```python
from build123d import *

# Parameters (mm, degrees)
SKETCH1_W             = 27
SKETCH1_H             = 27
SKETCH1_W_2           = 21
SKETCH1_H_2           = 21
BOSS_EXTRUDE1_DEPTH   = 70
BOSS_EXTRUDE1_2_DEPTH = 70
SKETCH2_W             = 120
SKETCH2_H             = 25
BOSS_EXTRUDE2_DEPTH   = 10
SKETCH3_W             = 3
SKETCH3_H             = 25
BOSS_EXTRUDE3_DEPTH   = 27
SKETCH4_R             = 2.15
CUT_EXTRUDE1_DEPTH    = 38


with BuildPart() as part:
    # Sketch1 → Boss-Extrude1 (new body)
    with BuildSketch(Plane(origin=(0, 0, 0), x_dir=(1, 0, 0), z_dir=(0, 1, 0))):
        with Locations((13.5, 13.5)):
            Rectangle(SKETCH1_W, SKETCH1_H)
        with Locations((13.5, 13.5)):
            Rectangle(SKETCH1_W_2, SKETCH1_H_2, mode=Mode.SUBTRACT)
    extrude(amount=BOSS_EXTRUDE1_DEPTH)



with BuildPart() as body_2:
    # Sketch1 → Boss-Extrude1 2 (new body)
    with BuildSketch(Plane(origin=(0, 0, 0), x_dir=(1, 0, 0), z_dir=(0, 1, 0))):
        with Locations((-16.5, 13.5)):
            Rectangle(SKETCH1_W, SKETCH1_H)
        with Locations((-16.5, 13.5)):
            Rectangle(SKETCH1_W_2, SKETCH1_H_2, mode=Mode.SUBTRACT)
    extrude(amount=BOSS_EXTRUDE1_2_DEPTH)


with BuildPart() as part_1:
    add(part.part)

    add(body_2.part)  # Boss-Extrude2 merges body 2
    # Sketch2 → Boss-Extrude2 (add)
    with BuildSketch(Plane.XY):
        with Locations((-2, 35)):
            Rectangle(SKETCH2_W, SKETCH2_H)
    extrude(amount=BOSS_EXTRUDE2_DEPTH)

    # Sketch3 → Boss-Extrude3 (add)
    with BuildSketch(Plane(origin=(0, 0, -27), x_dir=(-1, 0, 0), z_dir=(0, 0, -1))):
        with Locations((1.5, 35)):
            Rectangle(SKETCH3_W, SKETCH3_H)
    extrude(amount=-BOSS_EXTRUDE3_DEPTH)

    # Sketch4 → Cut-Extrude1 (cut, through all)
    with BuildSketch(Plane(origin=(0, 0, -27), x_dir=(-1, 0, 0), z_dir=(0, 0, -1))):
        with Locations((-13.5, 60)):
            Circle(SKETCH4_R)
        with Locations((16.5, 60)):
            Circle(SKETCH4_R)
        with Locations((-13.5, 10)):
            Circle(SKETCH4_R)
        with Locations((16.5, 10)):
            Circle(SKETCH4_R)
    extrude(amount=-CUT_EXTRUDE1_DEPTH, mode=Mode.SUBTRACT)


solid = part_1.part
```
Model file for the job. Use its own axes, mm. A direction names the side the tool comes from. Coordinates: 2 decimals unless noted, no trailing zeros. Loops run counter-clockwise (first coordinate to the right, second up) from the corner with the lowest first, then second, coordinate; pieces in that order, holes last. Notation, with made-up numbers: (51, 79.25) -> (77, 79.25) arc R23 cw to (77, 107.25) -> close; hole circle Ø5 at (-31, 65). An arc over 180 degrees is marked (long way). Answer as a JSON object with one key per item and string values.
Q1. 3-axis set-ups, long thin cutter, end or side, ignore diameter. For faces 1 (the flat face through (-17, 35, -24)), 2 (the flat face through (0, 11, -13)), 3 (the flat face through (0, 59, -13)): which of +Z, -Z, +X, -X, +Y, -Y reach the whole face in a straight line?
Report:
{"face 1": "+Y, -Y", "face 2": "+Z, -Z, -Y", "face 3": "+Z, -Z, +Y"}
Q2. Flat gauge pins, fed straight in: P1, Ø10.5, axis at y = 35, z = -10.5, coming from the -X side; P2, Ø7, axis at y = 55, z = -10.5, coming from the +X side; P3, Ø3.5, axis at x = -16.5, y = 10, coming from the +Z side; P4, Ø11, axis at x = 16.5, y = 53.5, coming from the +Z side. Where does each tip first touch, or does it go through?
Report:
{"P1": "stops at x = -30", "P2": "stops at x = 27", "P3": "passes through", "P4": "stops at z = 0"}
Q3. Pull direction Z, two halves, no side cores. Call faces 4 (the flat face through (13, 35, -3)), 5 (the flat face through (-2, 47.5, 4)), 6 (the flat face through (-27, 35, -13)): released by +Z, released by -Z, zero draft, split by the parting line, or undercut.
Report:
{"face 4": "undercut", "face 5": "zero draft", "face 6": "undercut"}
Q4. Cut at C-C (y = 17). List the corners of the cut face in (x, z).
Report:
{"outline": "(-30, -27) -> (-3, -27) -> (-3, 0) -> (-30, 0) -> close; (0, -27) -> (27, -27) -> (27, 0) -> (0, 0) -> close; hole (-27, -24) -> (-6, -24) -> (-6, -3) -> (-27, -3) -> close; hole (3, -24) -> (24, -24) -> (24, -3) -> (3, -3) -> close"}
Q5. Cut at D-D (z = -19). List the corners of the cut face in (x, y), and give its area (3 significant figures).
Report:
{"outline": "(-30, 0) -> (-27, 0) -> (-27, 70) -> (-30, 70) -> close; (-6, 0) -> (-3, 0) -> (-3, 22.5) -> (0, 22.5) -> (0, 0) -> (3, 0) -> (3, 70) -> (0, 70) -> (0, 47.5) -> (-3, 47.5) -> (-3, 70) -> (-6, 70) -> close; (24, 0) -> (27, 0) -> (27, 70) -> (24, 70) -> close", "area": "915 mm2"}
Q6. Cut at A-A (x = 13.5). List the corners of the cut face in (y, z).
Report:
{"outline": "(0, -27) -> (7.85, -27) -> (7.85, -24) -> (0, -24) -> close; (0, -3) -> (7.85, -3) -> (7.85, 0) -> (0, 0) -> close; (12.15, -27) -> (57.85, -27) -> (57.85, -24) -> (12.15, -24) -> close; (12.15, -3) -> (57.85, -3) -> (57.85, 0) -> (47.5, 0) -> (47.5, 10) -> (22.5, 10) -> (22.5, 0) -> (12.15, 0) -> close; (62.15, -27) -> (70, -27) -> (70, -24) -> (62.15, -24) -> close; (62.15, -3) -> (70, -3) -> (70, 0) -> (62.15, 0) -> close"}
Q7. Probe probe 1 along X at (y, z) = (5, -17.5); probe 2 along Z at (x, y) = (11, 67); probe 3 along Z at (x, y) = (-16, 46). List the from-to ranges inside material, lowest first.
Report:
{"probe 1": "x = -30 to -27, -6 to -3, 0 to 3, 24 to 27", "probe 2": "z = -27 to -24, -3 to 0", "probe 3": "z = -27 to -24, -3 to 10"}
Q8. Cut at B-B (y = 10). State how many separate pieces and enclosed holes the cut face has, and give its area (3 significant figures).
Report:
{"separate pieces": "4", "enclosed holes": "0", "area": "524 mm2"}
